Autodesk Inventor part; units mm, degrees
ref_plane "YZ Plane" through (0, 0, 0) normal (1, 0, 0) x (0, 1, 0)
ref_plane "XZ Plane" through (0, 0, 0) normal (0, 1, 0) x (-1, 0, 0)
ref_plane "XY Plane" through (0, 0, 0) normal (0, 0, 1) x (1, 0, 0)
sketch "Szkic3" plane through (0, 0, 0) normal (0, 1, 0) x (-1, 0, 0)
  line L0 (0, 0) -> (10, 0)
  line L1 (10, 0) -> (10, -50)
  line L2 (10, -50) -> (0, -50)
  line L3 (0, -50) -> (0, 0)
  circle A0 centre (5, -5) radius 2.5
  arc A1 (10, -2.5) -> (0, -2.5) centre (5, -6.25) ccw
  line L4 (8, -50) -> (2, -50)
  line L5 (2, -50) -> (2, -10)
  line L6 (2, -10) -> (8, -10)
  line L7 (8, -10) -> (8, -50)
  line L8 (2, -10) -> (8, -16)
  line L9 (2, -10) -> (10.4853, -10) construction
  line L10 (8, -16) -> (8, -18)
  line L11 (8, -18) -> (2, -12)
  line L12 (2, -10) -> (2, -12)
  line L13 (8, -18) -> (8, -22)
  line L14 (2, -16) -> (8, -22)
  line L15 (8, -24) -> (2, -18)
  line L16 (8, -16) -> (8, -14)
  line L17 (8, -24) -> (8, -26)
  line L18 (2, -20) -> (8, -26)
  line L19 (8, -28) -> (2, -22)
  line L20 (8, -28) -> (8, -32)
  line L21 (2, -26) -> (8, -32)
  line L22 (8, -34) -> (2, -28)
  line L23 (8, -34) -> (8, -36)
  line L24 (2, -26) -> (8, -32)
  line L25 (8, -34) -> (2, -28)
  line L26 (8, -34) -> (8, -38)
  line L27 (2, -32) -> (8, -38)
  line L28 (8, -40) -> (2, -34)
  line L29 (8, -40) -> (8, -42)
  line L30 (2, -32) -> (8, -38)
  line L31 (8, -40) -> (2, -34)
  line L32 (8, -40) -> (8, -44)
  line L33 (2, -38) -> (8, -44)
  line L34 (8, -46) -> (2, -40)
  line L35 (8, -46) -> (8, -48)
  line L36 (2, -38) -> (8, -44)
  line L37 (8, -46) -> (2, -40)
  line L38 (8, -46) -> (8, -50)
  line L39 (8, -46) -> (8, -48)
  line L40 (8, -48) -> (2, -42)
  line L41 (2, -42) -> (2, -44)
  line L42 (2, -44) -> (8, -50)
  line L43 (7, -49) -> (2, -49)
  circle A2 centre (5, -5) radius 3.25
  dimension "d9" = 10
  dimension "d10" = 50
  dimension "d11" = 5
  dimension "d12" = 6
  dimension "d13" = 40
  dimension "d14" = 45
  dimension "d15" = 2
  dimension "d16" = 4
  dimension "d17" = 2
  dimension "d18" = 2
  dimension "d19" = 2
  dimension "d20" = 2
  dimension "d21" = 4
  dimension "d22" = 2
  dimension "d23" = 2
  dimension "d24" = 2
  dimension "d25" = 4
  dimension "d26" = 2
  dimension "d27" = 2
  dimension "d28" = 2
  dimension "d29" = 4
  dimension "d30" = 2
  dimension "d32" = 2
  dimension "d36" = 2
  dimension "d37" = 2
  dimension "d42" = 6.5
extrude "Wyciągnięcie proste2" add sketch "Szkic3" against normal blind 2 contours A1 L1 L2 L7 L6 L5 L3 | L5 L43 L42 L2 | L42 L5 L40 L7 | L34 L5 L33 L7 | L28 L5 L27 L7 | L5 L21 L7 L22 | L5 L18 L7 L19 | L5 L14 L7 L15 | L5 L8 L7 L11 | A2
ref_plane "Płaszczyzna konstrukcyjna1" through (0, 0, -50) normal (0, 0, -1) x (-1, 0, 0)
mirror "Odbij1" about plane through (0, 0, -50) normal (0, 0, -1) of "Wyciągnięcie proste2"
sketch "Szkic4" plane through (0, 0, 0) normal (0, 1, 0) x (1, 0, 0)
  line L0 (-7.5, 91.0504) -> (-2.5, 91.0504)
  line L1 (-2.5, 91.0504) -> (-2.5, 98.6571)
  line L2 (-2.5, 98.6571) -> (-7.5, 98.6571)
  line L3 (-7.5, 98.6571) -> (-7.5, 91.0504)
  point P0 (0, 0)
extrude "Wyciągnięcie proste3" cut sketch "Szkic4" against normal blind 2
sketch "Szkic5" plane through (0, 0, 0) normal (0, 1, 0) x (1, 0, 0)
  line L0 (-10, 2.5) -> (-10, 97.5)
  line L1 (-10, 97.5) -> (-10, 67.5)
  line L2 (-10, 67.5) -> (-13, 67.5)
  line L3 (-13, 67.5) -> (-13, 97.5)
  line L4 (-13, 97.5) -> (-10, 97.5)
  arc A0 (0, 97.5) -> (-10, 97.5) centre (-5, 93.75) ccw
  line L5 (-5, 100) -> (-5, 49.8742)
  line L6 (-5, 100) -> (45.1258, 100) construction
  line L7 (-13, 67.5) -> (-10, 62.3038)
  line L8 (-13, 67.5) -> (-7, 67.5) construction
  line L9 (-10, 62.3038) -> (-10, 67.5)
  line L10 (0, 2.5) -> (0, 97.5)
  line L11 (0, 67.5) -> (3, 67.5)
  line L12 (3, 67.5) -> (3, 97.5)
  line L13 (3, 97.5) -> (0, 97.5)
  line L14 (3, 67.5) -> (0, 62.3038)
  arc A1 (3, 97.5) -> (-13, 97.5) centre (-5, 94.4495) ccw
  point P0 (0, 0)
  dimension "d43" = 30
  dimension "d44" = 3
  dimension "d45" = 90
  dimension "d46" = 60
extrude "Wyciągnięcie proste4" add sketch "Szkic5" against normal blind 2
sketch "Szkic6" plane through (0, 0, 0) normal (0, 1, 0) x (1, 0, 0)
  line L0 (-10, 62.3038) -> (-10, 2.5)
  line L1 (-10, 62.3038) -> (-10, 97.356)
  line L2 (-10, 97.356) -> (0, 97.356)
  line L3 (0, 97.356) -> (0, 62.3038)
  line L4 (0, 62.3038) -> (-10, 62.3038)
  point P0 (0, 0)
extrude "Wyciągnięcie proste5" cut sketch "Szkic6" against normal blind 2
sketch "Szkic7" plane through (0, 0, 0) normal (0, 1, 0) x (1, 0, 0)
  line L0 (-10, 62.3038) -> (-8, 62.3038)
  line L1 (-10, 62.3038) -> (-10, 67.4287)
  line L2 (-10, 62.3038) -> (-10, 97.356)
  line L3 (-10, 67.4287) -> (0, 67.4287)
  line L4 (0, 62.3038) -> (0, 97.356)
  line L5 (0, 62.3038) -> (0, 67.4287)
  line L6 (0, 62.3038) -> (-2, 62.3038)
  line L7 (-10, 2.5) -> (-10, 62.3038)
  line L8 (0, 62.3038) -> (-10, 62.3038)
  line L9 (-10, 62.3038) -> (-10, 61.2351)
  line L10 (-10, 61.2351) -> (0, 61.2351)
  line L11 (0, 61.2351) -> (0, 62.3038)
  line L12 (-10, 61.2351) -> (0, 61.2351)
  line L13 (0, 2.5) -> (0, 62.3038)
  line L14 (0, 61.2351) -> (0, 67.4287)
  line L15 (0, 67.4287) -> (-10, 67.4287)
  line L16 (-10, 61.2351) -> (-10, 67.4287)
  point P0 (0, 0)
extrude "Wyciągnięcie proste6" add sketch "Szkic7" against normal blind 2
sketch "Szkic8" plane through (0, 0, 0) normal (0, 1, 0) x (1, 0, 0)
  line L0 (-7.5, 97.356) -> (-10, 97.356)
  line L1 (-10, 97.356) -> (-11, 97.356)
  line L2 (-11, 97.356) -> (-11, 67.4287)
  line L3 (-11, 67.4287) -> (-10, 67.4287)
  line L4 (-10, 67.4287) -> (-10, 97.356)
  line L5 (0, 97.356) -> (1, 97.356)
  line L6 (1, 97.356) -> (1, 67.4287)
  line L7 (1, 67.4287) -> (0, 67.4287)
  line L8 (0, 67.4287) -> (0, 97.356)
  line L9 (-11, 67.4287) -> (1, 67.4287)
  line L10 (1, 67.4287) -> (1, 72.7222)
  line L11 (1, 72.7222) -> (-11, 72.7222)
  line L12 (-11, 72.7222) -> (-11, 67.4287)
  point P0 (0, 0)
  point P1 (0, 72.7222)
  point P2 (-10, 72.7222)
  dimension "d53" = 1
  dimension "d54" = 1
extrude "Wyciągnięcie proste7" cut sketch "Szkic8" against normal blind 2 contours L4 L11 L2 L1 | L8 L5 L6 L11
sketch "Szkic9" plane through (0, 0, 0) normal (0, 1, 0) x (1, 0, 0)
  line L0 (-10, 72.7222) -> (0, 72.7222)
  line L1 (0, 72.7222) -> (0, 67.3617)
  line L2 (0, 67.3617) -> (-10, 67.3617)
  line L3 (-10, 67.3617) -> (-10, 72.7222)
  point P0 (0, 0)
extrude "Wyciągnięcie proste8" add sketch "Szkic9" against normal blind 2
sketch "Szkic10" plane through (0, 0, 0) normal (0, 1, 0) x (1, 0, 0)
  point P0 (0, 0)
split "Podział1" plane through (0, 0, -50) removes the side toward (0, 0, -1)
sketch "Szkic11" plane through (0, 0, 0) normal (0, 1, 0) x (1, 0, 0)
  line L0 (-10, 2.5) -> (-10, 50)
  line L1 (-10, 50) -> (0, 50)
  line L2 (0, 50) -> (0, 100)
  line L3 (0, 100) -> (-10, 100)
  line L4 (-10, 100) -> (-10, 50)
  line L5 (-10, 100) -> (0, 100)
  line L6 (0, 100) -> (0, 124.634)
  line L7 (0, 124.634) -> (-10, 124.634)
  line L8 (-10, 124.634) -> (-10, 100)
  line L9 (-10, 124.634) -> (-11, 124.634)
  line L10 (-11, 124.634) -> (-11, 100)
  line L11 (-11, 100) -> (-10, 100)
  line L12 (-10, 100) -> (-10, 124.634)
  line L13 (0, 124.634) -> (1, 124.634)
  line L14 (1, 124.634) -> (1, 100)
  line L15 (1, 100) -> (0, 100)
  line L16 (0, 100) -> (0, 124.634)
  line L17 (-11, 100) -> (-9, 100) construction
  line L18 (1, 100) -> (3, 100) construction
  line L19 (-11, 124.634) -> (1, 124.634)
  line L20 (1, 124.634) -> (1, 126.634)
  line L21 (1, 126.634) -> (-11, 126.634)
  line L22 (-11, 126.634) -> (-11, 124.634)
  line L23 (-11, 100) -> (-12, 100)
  line L24 (-12, 100) -> (-12, 126.634)
  line L25 (-12, 126.634) -> (-11, 126.634)
  line L26 (-11, 126.634) -> (-11, 100)
  line L27 (1, 126.634) -> (2, 126.634)
  line L28 (2, 126.634) -> (2, 100)
  line L29 (2, 100) -> (1, 100)
  line L30 (1, 100) -> (1, 126.634)
  line L31 (-12, 100) -> (-10, 96.5359)
  line L32 (-12, 100) -> (-8, 100) construction
  line L33 (2, 100) -> (0, 96.5359)
  line L34 (2, 100) -> (6, 100) construction
  line L35 (-10, 124.634) -> (-10.5, 124.634)
  line L36 (-10.5, 124.634) -> (-10.5, 100)
  line L37 (0.5, 100) -> (0.5, 124.634)
  line L38 (0.75, 100) -> (0.75, 124.634)
  line L39 (-11, 100) -> (-10.75, 100)
  line L40 (-10.75, 100) -> (-10.75, 124.634)
  point P0 (0, 0)
  dimension "d59" = 10
  dimension "d60" = 50
  dimension "d61" = 10
  dimension "d62" = 24.634
  dimension "d63" = 1
  dimension "d64" = 1
  dimension "d67" = 2
  dimension "d68" = 1
  dimension "d69" = 1
  dimension "d70" = 60
  dimension "d71" = 120
  dimension "d90" = 0.5
  dimension "d107" = 0.25
extrude "Wyciągnięcie proste9" add sketch "Szkic11" against normal blind 2 contours L4 L3 L2 L1 | L31 L23 L11 L4 | L2 L15 L29 L33 | L24 L25 L22 L10 L23 | L29 L14 L20 L27 L28 | L9 L22 L21 L20 L13 L7
sketch "Szkic12" plane through (0, 0, 0) normal (0, 1, 0) x (1, 0, 0)
  line L0 (-8, 51.0298) -> (-2, 51.0298)
  line L1 (-2, 51.0298) -> (-2, 96.6875)
  line L2 (-2, 96.6875) -> (-8, 96.6875)
  line L3 (-8, 96.6875) -> (-8, 51.0298)
  line L4 (-8, 51.0298) -> (-2, 54.4939)
  line L5 (-8, 51.0298) -> (-1.0718, 51.0298) construction
  line L6 (-2, 54.4939) -> (-2, 59.4939)
  line L7 (-2, 59.4939) -> (-8, 56.0298)
  line L8 (-8, 51.0298) -> (-8, 56.0298)
  line L9 (-8, 56.0298) -> (-8, 61.0298)
  line L10 (-8, 61.0298) -> (-2, 64.4939)
  line L11 (-2, 64.4939) -> (-2, 69.4939)
  line L12 (-2, 69.4939) -> (-8, 66.0298)
  line L13 (-8, 61.0298) -> (-8, 66.0298)
  line L14 (-8, 66.0298) -> (-2, 69.4939)
  line L15 (-2, 74.4939) -> (-8, 71.0298)
  line L16 (-8, 76.0298) -> (-2, 79.4939)
  line L17 (-2, 84.4939) -> (-8, 81.0298)
  line L18 (-8, 71.0298) -> (-2, 74.4939)
  line L19 (-2, 79.4939) -> (-8, 76.0298)
  line L20 (-8, 81.0298) -> (-2, 84.4939)
  line L21 (-2, 89.4939) -> (-8, 86.0298)
  line L22 (-8, 76.0298) -> (-2, 79.4939)
  line L23 (-2, 84.4939) -> (-8, 81.0298)
  line L24 (-8, 86.0298) -> (-2, 89.4939)
  line L25 (-2, 94.4939) -> (-8, 91.0298)
  point P0 (0, 0)
  dimension "d74" = 30
  dimension "d75" = 5
  dimension "d76" = 5
  dimension "d77" = 5
  dimension "d78" = 5
  dimension "d79" = 5
  dimension "d80" = 5
  dimension "d81" = 5
  dimension "d82" = 5
  dimension "d83" = 5
  dimension "d84" = 5
  dimension "d85" = 5
  dimension "d86" = 5
extrude "Wyciągnięcie proste10" cut sketch "Szkic12" against normal blind 2 contours L3 L7 L1 L4 | L3 L12 L1 L10 | L3 L16 L1 L15 | L3 L21 L1 L17 | L3 L2 L1 L25
sketch "Szkic14" plane through (0, 0, 0) normal (0, 1, 0) x (1, 0, 0)
  arc A0 (5, 2.5) -> (15, 2.5) centre (10, 6.2465) ccw
  circle A1 centre (10, 5) radius 2.5
  line L0 (5, 2.5) -> (5, 5)
  line L1 (15, 2.5) -> (15, 5)
  line L2 (5, 5) -> (10, 104.8749)
  line L3 (10, 104.8749) -> (15, 5)
  line L4 (5.1827, 8.65) -> (14.8173, 8.65)
  line L5 (6.9979, 8.65) -> (12.6647, 8.65) construction
  line L6 (5.1827, 8.65) -> (7.1827, 8.65)
  line L7 (14.8173, 8.65) -> (12.8173, 8.65)
  line L8 (12.8173, 8.65) -> (9.8313, 56.0603)
  line L9 (9.8313, 56.0603) -> (7.1827, 8.65)
  line L10 (7.2581, 10) -> (12.7322, 10)
  point P0 (0, 0)
  dimension "d91" = 10
  dimension "d92" = 5
  dimension "d93" = 100
  dimension "d103" = 2
  dimension "d104" = 2
extrude "Wyciągnięcie proste11" add sketch "Szkic14" against normal blind 2 contours L0 L2 L4 L3 L1 A0 | L2 L3 L4 L8 L9 | L9 L10 L8 L4
sketch "Szkic15" plane through (0, 0, 0) normal (0, 1, 0) x (1, 0, 0)
  line L0 (-8, 91.0298) -> (-8, 96.6875)
  line L1 (-2, 10) -> (-8, 10)
  line L2 (-8, 96.6875) -> (-2, 96.6875)
  line L3 (-2, 96.6875) -> (-2, 10)
  line L4 (-2, 10) -> (-8, 10)
  line L5 (-8, 10) -> (-8, 96.6875)
  point P0 (0, 0)
extrude "Wyciągnięcie proste12" cut sketch "Szkic15" against normal blind 2
sketch "Szkic17" plane through (0, 0, 0) normal (0, 1, 0) x (1, 0, 0)
  line L0 (-2, 96.6875) -> (-8, 96.6875)
  line L1 (-8, 96.6875) -> (-8.5, 96.6875)
  line L2 (-8.5, 96.6875) -> (-7.5, 96.6875)
  line L3 (-2, 96.6875) -> (-2.5, 96.6875)
  line L4 (-2.5, 96.6875) -> (-1.5, 96.6875)
  line L5 (-8, 9.9943) -> (-8.5, 9.9943)
  line L6 (-8.5, 9.9943) -> (-7.5, 9.9943)
  line L7 (-2, 10) -> (-8, 10)
  line L8 (-2, 10) -> (-1.5, 10)
  line L9 (-1.5, 10) -> (-2.5, 10)
  line L10 (-1.5, 10) -> (-7.5, 96.6875)
  line L11 (-8.5, 96.6875) -> (-2.5, 10)
  line L12 (-7.5, 9.9943) -> (-1.5, 96.6875)
  line L13 (-2.5, 96.6875) -> (-8.5, 9.9943)
  point P0 (0, 0)
  point P1 (-4.9999, 60.5665)
  point P2 (-5.4999, 53.3423)
  point P3 (-4.9999, 46.1181)
  point P4 (-4.4999, 53.3423)
  dimension "d121" = 0.5
  dimension "d122" = 1
  dimension "d123" = 0.5
  dimension "d124" = 1
  dimension "d125" = 0.5
  dimension "d126" = 1
  dimension "d127" = 0.5
  dimension "d128" = 1
extrude "Wyciągnięcie proste14" add sketch "Szkic17" against normal blind 2 contours L4 L12 L10 L13 L0 | L10 L13 L11 L1 L0 | L10 L12 L11 L13 | L10 L8 L7 L11 L12 | L11 L12 L6 L5 L13
ref_plane "Płaszczyzna konstrukcyjna5" through (3.75, 0, -2.5) normal (-1, 0, 0) x (0, -1, 0)
ref_plane "Płaszczyzna konstrukcyjna4" through (0, 0, -2.5) normal (-1, 0, 0) x (0, -1, 0)
split "Podział2" plane through (3.75, 0, -2.5) removes the side toward (-1, 0, 0)
split "Podział3" plane through (3.75, 0, -2.5) removes the side toward (-1, 0, 0)
sketch "Szkic18" plane through (3.75, 0, -2.5) normal (-1, 0, 0) x (0, -1, 0)
  line L0 (-7.6237, -125.0024) -> (12.1257, -125.0024)
  line L1 (12.1257, -125.0024) -> (12.1257, 3.8459)
  line L2 (12.1257, 3.8459) -> (-7.6237, 3.8459)
  line L3 (-7.6237, 3.8459) -> (-7.6237, -125.0024)
  point P0 (0, 2.5)
extrude "Wyciągnięcie proste15" cut sketch "Szkic18" along normal blind 70
properties part number "arm_v2(arm-point)"
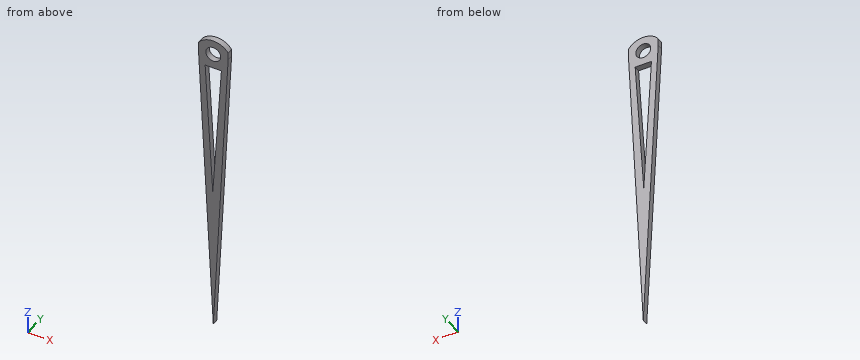
For this review, take the finished solid that the model builds, in its own axes (mm). Round coordinates to 2 decimals unless told otherwise and drop trailing zeros. Loops run counter-clockwise (first coordinate to the right, second up) from the corner with the lowest first, then second, coordinate; pieces in that order, holes last.
(1) We need section A-A (z = -32.5). Give the boundary of the cut face in (x, y).
Returned:
outline: (6.38, -2) - (8.52, -2) - (8.52, 0) - (6.38, 0) - close; (11.32, -2) - (13.62, -2) - (13.62, 0) - (11.32, 0) - close
(2) We need section C-C (z = -44). Give the boundary of the cut face in (x, y), plus the area to 3 significant figures.
Returned:
outline: (6.95, -2) - (9.16, -2) - (9.16, 0) - (6.95, 0) - close; (10.59, -2) - (13.05, -2) - (13.05, 0) - (10.59, 0) - close
area: 9.32 mm2
(3) We need section D-D (z = -77.5). Give the boundary of the cut face in (x, y), plus the area to 3 significant figures.
Returned:
outline: (8.63, -2) - (11.37, -2) - (11.37, 0) - (8.63, 0) - close
area: 5.48 mm2
(4) We need section B-B (y = -0.75). Give the boundary of the cut face in (x, z).
Returned:
outline: (5, -5) - (10, -104.87) - (15, -5) - (15, -2.5) arc R6.25 ccw to (5, -2.5) - close; hole (7.26, -10) - (9.83, -56.06) - (12.73, -10) - close; hole circle Ø5 at (10, -5)
(5) Wall thickness on line 1 along X through (y, z) = (-1.1, -5); line 2 along X through (y, z) = (-0.95, -38); line 3 along X through (y, z) = (-0.5, -74): over which ranges is each line inside the solid? List them lowest first.
Returned:
line 1: x = 5 to 7.5, 12.5 to 15
line 2: x = 6.65 to 8.82, 10.97 to 13.35
line 3: x = 8.45 to 11.55
(6) Clearance check with a flat-ended pin moving along its axis: P1, Ø1, axis at y = -1, z = -94, coming from the +X side. State where the tip first meets the part, or that it passes through.
Returned:
P1: stops at x = 10.57
